Build history of the part. All positions in model axes, mm. Face numbers are marked on the shaded views. A direction names the side the tool comes from. Give positions to 0.01 mm unless a question says otherwise; leave off trailing zeros. Loops run counter-clockwise (first coordinate to the right, second up) from the corner with the lowest first, then second, coordinate; pieces in that order, holes last. Notation, with made-up numbers: M 59,58.5 L 66,58.5 A22 cw 66,79.5 Z; hole C 9,38.25 d2. An arc over 180 degrees is marked long. Answer in a Markdown table with one row per item. Add a question column.
```python
from build123d import *

# Parameters (mm, degrees)
SKETCH1_W           = 40.132
SKETCH1_H           = 19.9136
BOSS_EXTRUDE1_DEPTH = 8.7122
SHELL1_T            = -1.7145
SKETCH3_R           = 3.683
BOSS_EXTRUDE2_DEPTH = 2.54
SKETCH4_R           = 2.54
CUT_EXTRUDE2_DEPTH  = 3.048
SKETCH8_R           = 1.778
BOSS_EXTRUDE5_DEPTH = 6.9977
SKETCH7_R           = 1.016
CUT_EXTRUDE5_DEPTH  = 8.7122
CHAMFER1_SIZE       = 2.3876
CHAMFER1_SIZE_2     = 1.27
SKETCH2_R           = 4.567425491
CUT_EXTRUDE6_DEPTH  = 1.016
SKETCH10_W          = 40.259
SKETCH10_H          = 19.9136
CUT_EXTRUDE7_DEPTH  = 0.6604
SKETCH11_W          = 5.08
SKETCH11_H          = 4.572
CUT_EXTRUDE8_DEPTH  = 1.7145
SKETCH12_R          = 8.5725
CUT_EXTRUDE9_DEPTH  = 6.9977


with BuildPart() as part:
    # Sketch1 → Boss-Extrude1 (new body)
    with BuildSketch(Plane(origin=(0, 0, 0), x_dir=(1, 0, 0), z_dir=(0, 1, 0))):
        Rectangle(SKETCH1_W, SKETCH1_H)
    extrude(amount=BOSS_EXTRUDE1_DEPTH)

    # Shell1
    shell1_openings = [part.faces().sort_by_distance(p)[0] for p in [
        (0, 0, 0),
    ]]
    offset(amount=SHELL1_T, openings=shell1_openings, kind=Kind.INTERSECTION)

    # Sketch3 → Boss-Extrude2 (add)
    with BuildSketch(Plane(origin=(0, 8.7122, 0), x_dir=(1, 0, 0), z_dir=(0, 1, 0))):
        with Locations(Location((10.2235, 0, 0), (0, 0, 90))):
            Circle(SKETCH3_R)
    extrude(amount=BOSS_EXTRUDE2_DEPTH)

    # Sketch4 → Cut-Extrude2 (cut)
    with BuildSketch(Plane(origin=(0, 11.2522, 0), x_dir=(1, 0, 0), z_dir=(0, 1, 0))):
        with Locations(Location((10.2235, 0, 0), (0, 0, 270))):
            Circle(SKETCH4_R)
    extrude(amount=-CUT_EXTRUDE2_DEPTH, mode=Mode.SUBTRACT)

    # Sketch8 → Boss-Extrude5 (add)
    with BuildSketch(Plane(origin=(0, 0, 0), x_dir=(-1, 0, 0), z_dir=(0, -1, 0))):
        with Locations((18.288, 8.1788)):
            Circle(SKETCH8_R)
        with Locations((-18.288, 8.1788)):
            Circle(SKETCH8_R)
        with Locations((18.288, -8.1788)):
            Circle(SKETCH8_R)
        with Locations((-18.288, -8.1788)):
            Circle(SKETCH8_R)
    extrude(amount=-BOSS_EXTRUDE5_DEPTH)

    # Sketch7 → Cut-Extrude5 (cut)
    with BuildSketch(Plane(origin=(0, 0, 0), x_dir=(-1, 0, 0), z_dir=(0, -1, 0))):
        with Locations(Location((18.0848, 7.9756, 0), (0, 0, 90))):
            Circle(SKETCH7_R)
        with Locations(Location((-18.0848, 7.9756, 0), (0, 0, 90))):
            Circle(SKETCH7_R)
        with Locations(Location((18.0848, -7.9756, 0), (0, 0, 90))):
            Circle(SKETCH7_R)
        with Locations(Location((-18.0848, -7.9756, 0), (0, 0, 90))):
            Circle(SKETCH7_R)
    extrude(amount=-CUT_EXTRUDE5_DEPTH, mode=Mode.SUBTRACT)

    # Chamfer1
    # the kernel refuses this chamfer: 2.3876, 1.27 mm, written as the material it takes off along each edge
    with BuildSketch(Plane(origin=(20.066, 8.7122, 16.137611711), x_dir=(0.018140787758026848, -0.9998354423701522, 0), z_dir=(0, 0, -1))) as chamfer1_piece_1:
        Polygon((CHAMFER1_SIZE * 0.99983544237, CHAMFER1_SIZE * 0.018140787758), (-CHAMFER1_SIZE_2 * 0.018140787758, CHAMFER1_SIZE_2 * 0.99983544237), (0, 0), align=None)
    extrude(amount=32.275223423, mode=Mode.SUBTRACT)
    with BuildSketch(Plane(origin=(26.246811711, 8.7122, -9.9568), x_dir=(0, -0.9998354423701524, -0.01814078775802685), z_dir=(-1, 0, 0))) as chamfer1_piece_2:
        Polygon((CHAMFER1_SIZE * 0.99983544237, CHAMFER1_SIZE * 0.018140787758), (-CHAMFER1_SIZE_2 * 0.018140787758, CHAMFER1_SIZE_2 * 0.99983544237), (0, 0), align=None)
    extrude(amount=52.493623423, mode=Mode.SUBTRACT)
    with BuildSketch(Plane(origin=(-20.066, 8.7122, -16.137611711), x_dir=(0.9979501613334688, 0.06399590216962081, 0), z_dir=(0, 0, 1))) as chamfer1_piece_3:
        Polygon((CHAMFER1_SIZE_2 * 0.997950161333, -CHAMFER1_SIZE_2 * 0.0639959021696), (-CHAMFER1_SIZE * 0.0639959021696, -CHAMFER1_SIZE * 0.997950161333), (0, 0), align=None)
    extrude(amount=32.275223423, mode=Mode.SUBTRACT)
    with BuildSketch(Plane(origin=(-26.246811711, 8.7122, 9.9568), x_dir=(0, 0.06399590216962081, -0.9979501613334687), z_dir=(1, 0, 0))) as chamfer1_piece_4:
        Polygon((CHAMFER1_SIZE_2 * 0.997950161333, -CHAMFER1_SIZE_2 * 0.0639959021696), (-CHAMFER1_SIZE * 0.0639959021696, -CHAMFER1_SIZE * 0.997950161333), (0, 0), align=None)
    extrude(amount=52.493623423, mode=Mode.SUBTRACT)

    # Sketch2 → Cut-Extrude6 (cut)
    with BuildSketch(Plane(origin=(0, 8.7122, 0), x_dir=(1, 0, 0), z_dir=(0, 1, 0))):
        with Locations((20.066, 9.9568)):
            Circle(SKETCH2_R)
        with Locations((-20.066, 9.9568)):
            Circle(SKETCH2_R)
        with Locations((-20.066, -9.9568)):
            Circle(SKETCH2_R)
        with Locations((20.066, -9.9568)):
            Circle(SKETCH2_R)
    extrude(amount=-CUT_EXTRUDE6_DEPTH, mode=Mode.SUBTRACT)

    # Sketch10 → Cut-Extrude7 (cut)
    with BuildSketch(Plane(origin=(0, 0, 0), x_dir=(-1, 0, 0), z_dir=(0, -1, 0))):
        with Locations((0.0635, 0)):
            Rectangle(SKETCH10_W, SKETCH10_H)
    extrude(amount=-CUT_EXTRUDE7_DEPTH, mode=Mode.SUBTRACT)

    # Sketch11 → Cut-Extrude8 (cut)
    with BuildSketch(Plane(origin=(20.066, 0, 0), x_dir=(0, 0, -1), z_dir=(1, 0, 0))):
        with Locations((0, 2.286)):
            Rectangle(SKETCH11_W, SKETCH11_H)
    extrude(amount=-CUT_EXTRUDE8_DEPTH, mode=Mode.SUBTRACT)

    # Sketch12 → Cut-Extrude9 (cut)
    with BuildSketch(Plane(origin=(0, 0, 0), x_dir=(-1, 0, 0), z_dir=(0, -1, 0))):
        with Locations((10.2997, 0)):
            Circle(SKETCH12_R)
    extrude(amount=-CUT_EXTRUDE9_DEPTH, mode=Mode.SUBTRACT)


solid = part.part
```
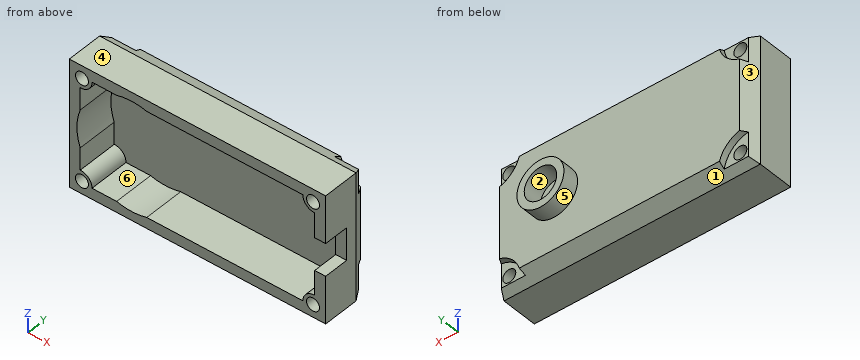
(1) Pin check, flat tips, straight feed: pin 1 (8.5 mm diameter, centred on x = 1.5, z = -3, fed in from -Y); pin 2 (1.9 mm diameter, centred on x = 17, z = 7.5, fed in from +Y); pin 3 (1.1 mm diameter, centred on x = -17.5, z = 8, fed in from +Y); pin 4 (1.8 mm diameter, centred on x = -18.08, z = 7.98, fed in from -Y). Stop position of each tip, or through.
(2) Tool access for the marked faces 4, 5 and 6: list every direction of +Z, -Z, +X, -X, +Y, -Y with a clear straight run to the whole face (end or side of a thin tool).
(3) Slice it at A-A, the plane x = 5. Give the cut face in (y, z), then the cut area to 3 significant figures.
(4) Slice it at C-C, the plane z = -2. Give the cut face in (x, y).
(5) Slice it at D-D, the plane x = -12. Give the cut face in (y, z).
(6) Slice it at B-B, the plane z = 0. Give the cut face in (x, y), then the cut area to 3 significant figures.
(7) Wall check: line 1 (Z direction, x = 8.5, y = 4.25); line 2 (X direction, y = 9.9, z = 0); line 3 (X direction, y = 5.75, z = -5.5). Give the ranges that are in metal, low to high.
(8) Pull direction X, two halves, no side cores. Call the marked faces 1, 2 and 3: +X half, -X half, draft (parallel to the pull), parting line (faces both ways), or undercut.
Solution:
| question | item | result |
|---|---|---|
| 1 | pin 1 | y = 7 |
| 1 | pin 2 | y = 8.71 |
| 1 | pin 3 | y = 7.7 |
| 1 | pin 4 | through |
| 2 | face 4 | +Z, +X, -X, +Y, -Y |
| 2 | face 5 | +Y |
| 2 | face 6 | -Y |
| 3 | outline | M 0.66,-9.96 L 6.32,-9.96 L 8.71,-8.69 L 8.71,8.69 L 6.32,9.96 L 0.66,9.96 L 0.66,8.24 L 7,8.24 L 7,-8.24 L 0.66,-8.24 Z |
| 3 | area | 52.8 mm^2 |
| 4 | outline | M -20.07,0.66 L -18.64,0.66 L -18.64,7 L 18.35,7 L 18.35,4.57 L 20.07,4.57 L 20.07,6.32 L 18.8,8.71 L 13.32,8.71 L 13.32,11.25 L 11.79,11.25 L 11.79,8.2 L 8.66,8.2 L 8.66,11.25 L 7.13,11.25 L 7.13,8.71 L -18.8,8.71 L -20.07,6.32 Z |
| 5 | outline | M 0.66,-9.96 L 6.32,-9.96 L 8.71,-8.69 L 8.71,8.69 L 6.32,9.96 L 0.66,9.96 L 0.66,8.4 L 7,8.4 L 7,-8.4 L 0.66,-8.4 Z |
| 6 | outline | M -20.07,0.66 L -18.87,0.66 L -18.87,7 L 18.35,7 L 18.35,4.57 L 20.07,4.57 L 20.07,6.32 L 18.8,8.71 L 13.91,8.71 L 13.91,11.25 L 12.76,11.25 L 12.76,8.2 L 7.68,8.2 L 7.68,11.25 L 6.54,11.25 L 6.54,8.71 L -18.8,8.71 L -20.07,6.32 Z |
| 6 | area | 80.7 mm^2 |
| 7 | line 1 | -9.96 to -8.24, 8.24 to 9.96 |
| 7 | line 2 | 6.54 to 7.68, 12.76 to 13.91 |
| 7 | line 3 | -20.07 to -18.35, 18.35 to 20.07 |
| 8 | face 1 | draft |
| 8 | face 2 | undercut |
| 8 | face 3 | -X half |
